Build history of the part. All positions in model axes, mm. Face numbers are marked on the shaded views. A direction names the side the tool comes from. Give positions to 0.01 mm unless a question says otherwise; leave off trailing zeros. Order: outer loops, then holes, each group sorted by start corner. A loop starts at its lowest first (then second) coordinate and runs counter-clockwise, first axis right, second up. Notation, with made-up numbers: (-32, -5) -> (-22, -5) arc R7 cw to (-22, 1) -> close; hole circle Ø4 at (15, 8). An arc over 180 degrees is marked (long way). Write item = value, one per line. Start each with the question number.
from build123d import *

# Parameters (mm, degrees)
SKETCH_1_R      = 1.5
EXTRUDE_2_DEPTH = 10


with BuildPart() as part:
    # 草图1 → 凸台-拉伸2 (new body)
    with BuildSketch(Plane(origin=(0, 0, 0), x_dir=(0, 0, -1), z_dir=(1, 0, 0))):
        with BuildLine():
            ThreePointArc((17.320508076, -10), (-1.743114855, -19.923893962), (-18.793852416, -6.840402867))
            Line((-18.793852416, -6.840402867), (-24.485520572, 8.797326871))
            ThreePointArc((-24.485520572, 8.797326871), (-24.06362866, 12.001914989), (-21.196596456, 13.494397531))
            Line((-21.196596456, 13.494397531), (-21.045218822, 13.494397531))
            ThreePointArc((-21.045218822, 13.494397531), (-20.53641173, 14.256780606), (-20, 15))
            Line((-20, 15), (-20, 15.803944373))
            Line((-20, 15.803944373), (-24.155954344, 19.087967936))
            ThreePointArc((-24.155954344, 19.087967936), (-28.049684886, 19.919774087), (-31.079320854, 17.336298731))
            ThreePointArc((-31.079320854, 17.336298731), (-35.972771838, 10.757774611), (-43.301092247, 7.081014883))
            ThreePointArc((-43.301092247, 7.081014883), (-46.36357592, 0.839616609), (-39.647678535, -0.957765092))
            ThreePointArc((-39.647678535, -0.957765092), (-30.443187857, 0.329762523), (-24.14010081, -6.500425592))
            ThreePointArc((-24.14010081, -6.500425592), (-3.247781267, -24.788140649), (21.650635095, -12.5))
            Line((21.650635095, -12.5), (37.127801325, 14.307238269))
            Line((37.127801325, 14.307238269), (38.323661657, 20.544349721))
            Line((38.323661657, 20.544349721), (37.457636253, 21.044349721))
            Line((37.457636253, 21.044349721), (32.797674306, 16.807238269))
            Line((32.797674306, 16.807238269), (17.320508076, -10))
        make_face()
        with Locations((-26.945927107, 15.557238269)):
            Circle(SKETCH_1_R, mode=Mode.SUBTRACT)
        with Locations((-42.266815969, 2.701486075)):
            Circle(SKETCH_1_R, mode=Mode.SUBTRACT)
    extrude(amount=EXTRUDE_2_DEPTH)


solid = part.part
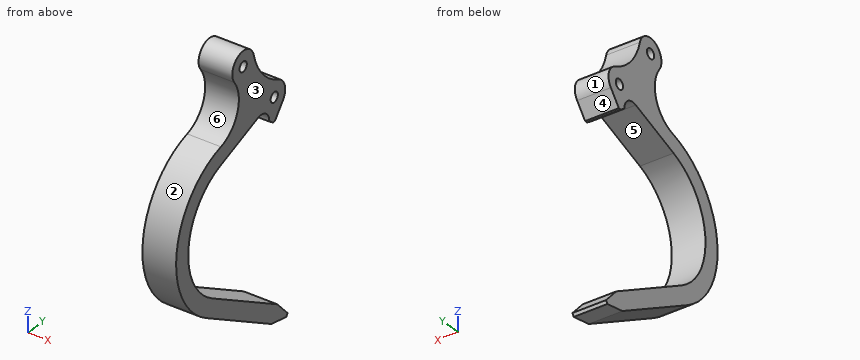
(1) Cut at A-A, the plane y = -17.5. Give the cut face in (x, z).
(2) Cut at B-B, the plane z = 26.5. Give the cut face in (x, y), plus the area to 3 significant figures.
(3) Wall check: line 1 (Z direction, x = 3, y = 3); line 2 (Z direction, x = 6.5, y = -16.5); line 3 (Z direction, x = 4, y = -4.5). Give the ranges that are in metal, low to high. Write a range as [from, to].
(4) Cut at D-D, the plane z = -9.5. Give the cut face in (x, y), plus the area to 3 significant figures.
(5) 3-axis set-ups, long thin cutter, end or side, ignore diameter. For the marked faces 4, 5 and 6: which of +Z, -Z, +X, -X, +Y, -Y reach the whole face in a straight line?
(6) Cut at C-C, the plane x = 7.5. Give the cut face in (y, z), plus the area to 3 significant figures.
(7) Mould opens along Z. For the marked faces 1, 2 and 3 say: released by +Z, released by -Z, zero draft, split by the parting line, or undercut.
(8) Flat gauge pins, fed straight in: P1, Ø4, axis at x = 1.5, z = 27, coming from the -Y side; P2, Ø5, axis at x = 5, z = -22, coming from the +Y side; P3, Ø4, axis at x = 9, y = -19, coming from the +Z side. Where does each tip first touch, or does it go through?
Results:
q1.outline = (0, -17.85) -> (10, -17.85) -> (10, -9.68) -> (0, -9.68) -> close; (0, 9.68) -> (10, 9.68) -> (10, 17.85) -> (0, 17.85) -> close
q2.outline = (0, -2.26) -> (10, -2.26) -> (10, 14.13) -> (0, 14.13) -> close; (0, 16.99) -> (10, 16.99) -> (10, 20.04) -> (0, 20.04) -> close
q2.area = 194 mm2
q3.line_1 = [-30.6, -24.83], [22.38, 40.8], [43.74, 46.76]
q3.line_2 = [-18.78, -11.3], [11.3, 18.78]
q3.line_3 = [-26.27, -20.5], [19.65, 24.92]
q4.outline = (0, -23.12) -> (10, -23.12) -> (10, -17.6) -> (0, -17.6) -> close
q4.area = 55.2 mm2
q5.face_4 = +X, -X, +Y
q5.face_5 = +X, -X
q5.face_6 = +X, -X, -Y
q6.outline = (-12.5, -21.65) -> (14.31, -37.13) -> (20.54, -38.32) -> (21.04, -37.46) -> (16.81, -32.8) -> (-10, -17.32) arc R20 cw to (-6.84, 18.79) -> (8.8, 24.49) arc R3.5 cw to (13.49, 21.2) -> (13.49, 21.05) arc R25 cw to (15, 20) -> (15.8, 20) -> (19.09, 24.16) arc R4.5 ccw to (17.34, 31.08) arc R17.75 cw to (7.08, 43.3) arc R4.5 ccw (long way) to (-0.96, 39.65) arc R10.02 cw to (-6.5, 24.14) arc R25 ccw to start; hole circle Ø3 at (2.7, 42.27); hole circle Ø3 at (15.56, 26.95)
q6.area = 774 mm2
q7.face_1 = undercut
q7.face_2 = split by the parting line
q7.face_3 = zero draft
q8.P1 = -4.34
q8.P2 = 2.44
q8.P3 = 18.33
